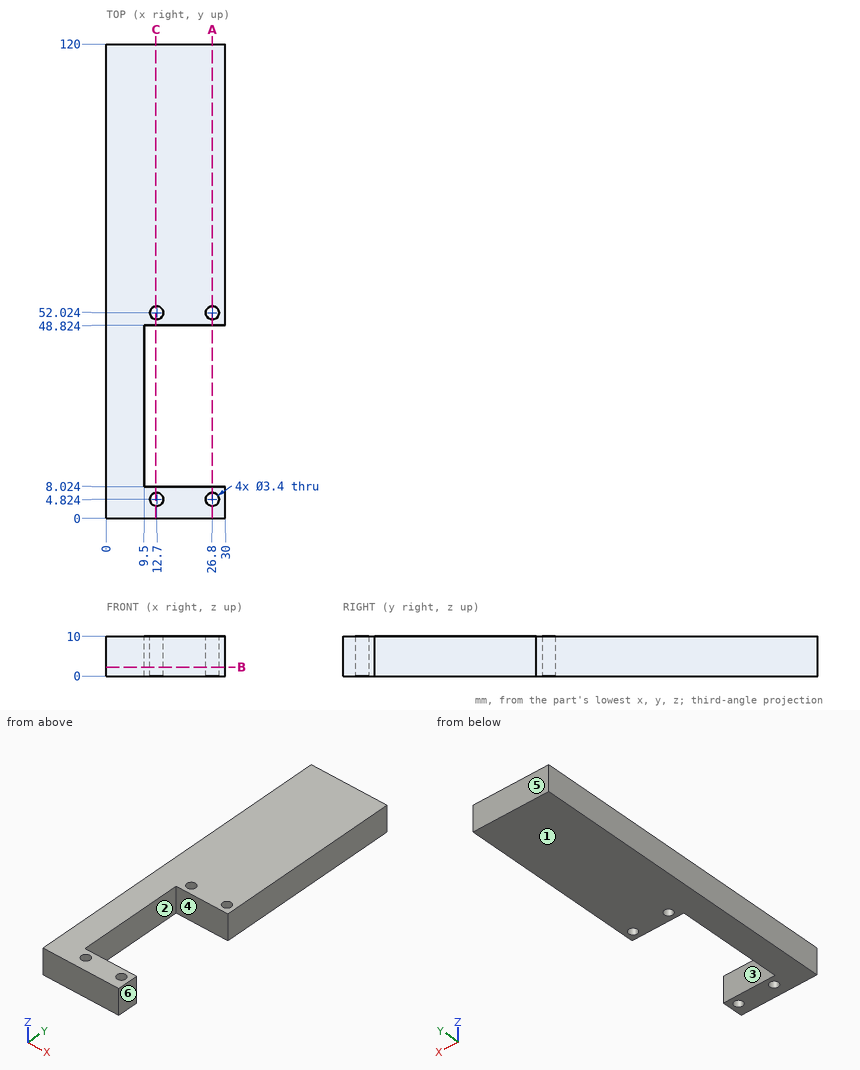
Study the drawing (mm; zero at the part's minimum x, y, z) and answer. A direction names the side the tool comes from. Give positions to 0.01 mm unless a question says otherwise; leave off trailing zeros. Loops run counter-clockwise (first coordinate to the right, second up) from the corner with the lowest first, then second, coordinate; pieces in that order, holes last. Notation, with made-up numbers: (-8.75, -5.75) - (23.25, -5.75) arc R19 cw to (23.25, 16.25) - close; hole circle Ø8 at (15.5, 50). An arc over 180 degrees is marked (long way). Answer in a Markdown table with one row per item. Add a question column.
Q1. The part is cut by section B-B (z = 2.25). Determine the outline of the cut face in (x, y), and give its area (3 significant figures).
Q2. A tool of negligible diameter and unlimited length cuts with its end or side. For the marked faces 1 and 2, from which of +Z, -Z, +X, -X, +Y, -Y can it reach the whole face along a straight path? Write none if from no direction.
Q3. Determine the mould class of the marked faces 3, 4, 5 and 6 for opening direction Y: released by +Y, released by -Y, zero draft, split by the parting line, or undercut.
Q4. The part is cut by section A-A (x = 26.8). Determine the outline of the cut face in (y, z), and give its area (3 significant figures).
Q5. Consider line 1 along Y through (x, z) = (12.7, 2.25); line 2 along Y through (x, z) = (15.25, 3); line 3 along Y through (x, z) = (26, 4.25). Determine where each line is inside the solid, lowest interval first.
Q6. The part is cut by section C-C (x = 12.5). Determine the outline of the cut face in (y, z) (1 decimal).
Solution:
| question | item | result |
|---|---|---|
| 1 | outline | (0, 0) - (30, 0) - (30, 8.02) - (9.5, 8.02) - (9.5, 48.82) - (30, 48.82) - (30, 120) - (0, 120) - close; hole circle Ø3.4 at (12.7, 4.82); hole circle Ø3.4 at (12.7, 52.02); hole circle Ø3.4 at (26.8, 4.82); hole circle Ø3.4 at (26.8, 52.02) |
| 1 | area | 2,730 mm² |
| 2 | face 1 | -Z, +X, -X, +Y, -Y |
| 2 | face 2 | +Z, -Z, +X |
| 3 | face 3 | undercut |
| 3 | face 4 | undercut |
| 3 | face 5 | released by +Y |
| 3 | face 6 | zero draft |
| 4 | outline | (0, 0) - (3.12, 0) - (3.12, 10) - (0, 10) - close; (6.52, 0) - (8.02, 0) - (8.02, 10) - (6.52, 10) - close; (48.82, 0) - (50.32, 0) - (50.32, 10) - (48.82, 10) - close; (53.72, 0) - (120, 0) - (120, 10) - (53.72, 10) - close |
| 4 | area | 724 mm² |
| 5 | line 1 | y = 0 to 3.12, 6.52 to 8.02, 48.82 to 50.32, 53.72 to 120 |
| 5 | line 2 | y = 0 to 8.02, 48.82 to 120 |
| 5 | line 3 | y = 0 to 3.32, 6.32 to 8.02, 48.82 to 50.52, 53.52 to 120 |
| 6 | outline | (0, 0) - (3.1, 0) - (3.1, 10) - (0, 10) - close; (6.5, 0) - (8, 0) - (8, 10) - (6.5, 10) - close; (48.8, 0) - (50.3, 0) - (50.3, 10) - (48.8, 10) - close; (53.7, 0) - (120, 0) - (120, 10) - (53.7, 10) - close |
